```python
from build123d import *

# Parameters (mm, degrees)
EXTRUDE_1_DEPTH   = 2.5
MM_1_D            = 3
CHAMFER_START     = -3
CHAMFER_1_DEPTH   = 6
CHAMFER_START_2   = -2.5
CHAMFER_1_2_DEPTH = 5


with BuildPart() as part:
    # 草图1 → 凸台-拉伸1 (new, symmetric)
    with BuildSketch(Plane.XY):
        Polygon((5, 0), (10, 0), (10, 5), (-10, 5), (-10, 0), (-5, 0), (-5, 1), (5, 1), align=None)
    extrude(amount=EXTRUDE_1_DEPTH, both=True)

    # 大小mm 暗销孔1 (through all)
    with Locations(Plane(origin=(0, 5, 0), x_dir=(1, 0, 0), z_dir=(0, 1, 0))):
        with Locations((-7.5, 0), (7.5, 0)):
            Hole(MM_1_D / 2)

    # 倒角1: read off the stored shape, not the designer's step
    # 倒角1 outline → 倒角1 (cut)
    with BuildSketch(Plane.XY.offset(CHAMFER_START)):
        Polygon((10, 5), (9, 5), (10, 4), align=None)
        Polygon((-10, 4), (-9, 5), (-10, 5), align=None)
    extrude(amount=CHAMFER_1_DEPTH, mode=Mode.SUBTRACT)

    # Chamfer 1 2 outline → Chamfer 1 2 (add)
    with BuildSketch(Plane.XY.offset(CHAMFER_START_2)):
        Polygon((5, 1), (4, 1), (5, 0), align=None)
        Polygon((-5, 0), (-4, 1), (-5, 1), align=None)
    extrude(amount=CHAMFER_1_2_DEPTH)


solid = part.part
```
Design review of the part built by this model. Coordinates are the model's own, in mm. A direction names the side the tool comes from. Round coordinates to 2 decimals unless told otherwise and drop trailing zeros. Order: outer loops, then holes, each group sorted by start corner. A loop starts at its lowest first (then second) coordinate and runs counter-clockwise, first axis right, second up. Notation, with made-up numbers: (5, -32.75) - (19, -32.75) arc R16 ccw to (19, -26.75) - close; hole circle Ø9 at (83.5, 38). An arc over 180 degrees is marked (long way). One line per question, with ' | ' between items.
Item 1: Take a section at A-A, the plane y = 0.5. Write out the cut boundary in (x, z), then the cut area to 3 significant figures.
Checks:
outline: (-10, -2.5) - (-4.5, -2.5) - (-4.5, 2.5) - (-10, 2.5) - close; (4.5, -2.5) - (10, -2.5) - (10, 2.5) - (4.5, 2.5) - close; hole circle Ø3 at (-7.5, 0); hole circle Ø3 at (7.5, 0) | area: 40.9 mm²
Item 2: Take a section at B-B, the plane x = -7.5. Write out the cut boundary in (y, z).
Checks:
outline: (0, -2.5) - (5, -2.5) - (5, -1.5) - (0, -1.5) - close; (0, 1.5) - (5, 1.5) - (5, 2.5) - (0, 2.5) - close
Item 3: Draft analysis for pull direction Z (two halves, no side actions). For faces 3 (the face through (-6, 2, 0)), 4 (the face through (9, 2, 0)), 5 (the face through (9.5, 4.5, 0)), 6 (the face through (0, 3, 2.5)), state which applies: +Z half, -Z half, draft (parallel to the pull), parting line (faces both ways), or undercut.
Checks:
face 3: undercut | face 4: undercut | face 5: draft | face 6: +Z half
Item 4: Wall thickness on line 1 (X direction, y = 1.8, z = 0.45); line 2 (X direction, y = 3.45, z = 1); line 3 (Z direction, x = 7.5, y = 1.05): over which ranges is each line inside the solid? List them lowest first. Write a range as [from, to].
Checks:
line 1: [-10, -8.93], [-6.07, 6.07], [8.93, 10] | line 2: [-10, -8.62], [-6.38, 6.38], [8.62, 10] | line 3: [-2.5, -1.5], [1.5, 2.5]
Item 5: Take a section at C-C, the plane z = -0.7. Write out the cut boundary in (x, y).
Checks:
outline: (-10, 0) - (-8.83, 0) - (-8.83, 5) - (-9, 5) - (-10, 4) - close; (-6.17, 0) - (-5, 0) - (-4, 1) - (4, 1) - (5, 0) - (6.17, 0) - (6.17, 5) - (-6.17, 5) - close; (8.83, 0) - (10, 0) - (10, 4) - (9, 5) - (8.83, 5) - close
Item 6: Machinability: for faces 1 (the face through (0, 1, 0)), 2 (the face through (0, 5, 0)), which of the approach directions +Z, -Z, +X, -X, +Y, -Y give a long, thin tool a straight path to every point of the face, cutting with its end or side? Answer none if there is none.
Checks:
face 1: +Z, -Z, -Y | face 2: +Z, -Z, +X, -X, +Y
Item 7: Take a section at D-D, the plane y = 4.2. Write out the cut boundary in (x, z), then the cut area to 3 significant figures.
Checks:
outline: (-9.8, -2.5) - (9.8, -2.5) - (9.8, 2.5) - (-9.8, 2.5) - close; hole circle Ø3 at (-7.5, 0); hole circle Ø3 at (7.5, 0) | area: 83.9 mm²
Item 8: For P1, Ø1, axis at x = -6.5, z = 2, coming from the -Y side; P2, Ø2.5, axis at x = -7.5, z = 0, coming from the +Y side; P3, Ø1.5, axis at x = 1.5, z = 0, coming from the -Y side, all flat-tipped, find the tip position at first contact; note any pin that passes through.
Checks:
P1: y = 0 | P2: through | P3: y = 1
